CAD build for the part. Positions are in the model's coordinates, mm. Round coordinates to 2 decimals unless told otherwise and drop trailing zeros. Order: outer loops, then holes, each group sorted by start corner. A loop starts at its lowest first (then second) coordinate and runs counter-clockwise, first axis right, second up. Notation, with made-up numbers: M 81.25,32 L 114.25,32 A5 cw 114.25,37 Z; hole C 57,29.25 d3. An arc over 180 degrees is marked long. Answer as a JSON object with one key per item and string values.
```python
from build123d import *

# Parameters (mm, degrees)
SKETCH1_W           = 15
SKETCH1_H           = 24
BOSS_EXTRUDE1_DEPTH = 4
SKETCH2_R           = 2.5
SKETCH2_R_2         = 1.6
CUT_EXTRUDE1_DEPTH  = 29.583211856
FILLET1_R           = 5


with BuildPart() as part:
    # Sketch1 → Boss-Extrude1 (new body)
    with BuildSketch(Plane(origin=(0, 0, 0), x_dir=(0, 0, -1), z_dir=(1, 0, 0))):
        with Locations((7.5, -12)):
            Rectangle(SKETCH1_W, SKETCH1_H)
    extrude(amount=BOSS_EXTRUDE1_DEPTH)

    # Sketch2 → Cut-Extrude1 (cut, through all)
    with BuildSketch(Plane(origin=(4, 0, 0), x_dir=(0, 0, -1), z_dir=(1, 0, 0))):
        with Locations((7.5, -20)):
            Circle(SKETCH2_R)
        with Locations((7.5, -4)):
            Circle(SKETCH2_R_2)
    extrude(amount=-CUT_EXTRUDE1_DEPTH, mode=Mode.SUBTRACT)

    # Fillet1
    fillet1_edges = [part.edges().sort_by_distance(p)[0] for p in [
        (2, 0, 0),
        (2, 0, -15),
        (2, -24, -15),
        (2, -24, 0),
    ]]
    fillet(fillet1_edges, radius=FILLET1_R)


solid = part.part
```
Item 1: Drop flat-ended pins along their axis: pin 1 Ø4.5 at (y, z) = (-20, -7.5) entering from -X; pin 2 Ø1 at (x, z) = (2.5, -11) entering from -Y. Give the stop position or say it passes through.
Worked answers:
{"pin 1": "passes through", "pin 2": "stops at y = -23.97"}
Item 2: Two-plate mould, pull along Y, no slides. Class faces 1 (the cylindrical face through (2.03, -2.92, -6.32)), 2 (the flat face through (2, 0, -7)), 3 (the cylindrical face through (2, -22, -1)), 4 (the flat face through (0, -12, -7)): released by +Y, released by -Y, zero draft, split by the parting line, or undercut.
Worked answers:
{"face 1": "undercut", "face 2": "released by +Y", "face 3": "released by -Y", "face 4": "zero draft"}
Item 3: Wall check: line 1 along Y through (x, z) = (1.2, -7.5); line 2 along Z through (x, y) = (1.75, -20.75); line 3 along Y through (x, z) = (1.4, -6.75). Give the ranges that are in metal, low to high. Write a range as [from, to].
Worked answers:
{"line 1": "y = [-24, -22.5], [-17.5, -5.6], [-2.4, 0]", "line 2": "z = [-14.68, -9.88], [-5.12, -0.32]", "line 3": "y = [-24, -22.38], [-17.62, -5.41], [-2.59, 0]"}
Item 4: Saw through at B-B on x = 1.05. List the corners of the cut face in (y, z), and give its area (3 significant figures).
Worked answers:
{"outline": "M -24,-10 A5 ccw -19,-15 L -5,-15 A5 ccw 0,-10 L 0,-5 A5 ccw -5,0 L -19,0 A5 ccw -24,-5 Z; hole C -20,-7.5 d5; hole C -4,-7.5 d3.2", "area": "311 mm2"}
Item 5: Saw through at C-C on y = -22. List the corners of the cut face in (x, z).
Worked answers:
{"outline": "M 0,-14 L 4,-14 L 4,-9 L 0,-9 Z; M 0,-6 L 4,-6 L 4,-1 L 0,-1 Z"}
Item 6: Saw through at D-D on y = -18.25. List the corners of the cut face in (x, z).
Worked answers:
{"outline": "M 0,-15 L 4,-15 L 4,-9.29 L 0,-9.29 Z; M 0,-5.71 L 4,-5.71 L 4,0 L 0,0 Z"}
Item 7: Saw through at A-A on z = -7.5. List the corners of the cut face in (x, y).
Worked answers:
{"outline": "M 0,-24 L 4,-24 L 4,-22.5 L 0,-22.5 Z; M 0,-17.5 L 4,-17.5 L 4,-5.6 L 0,-5.6 Z; M 0,-2.4 L 4,-2.4 L 4,0 L 0,0 Z"}
